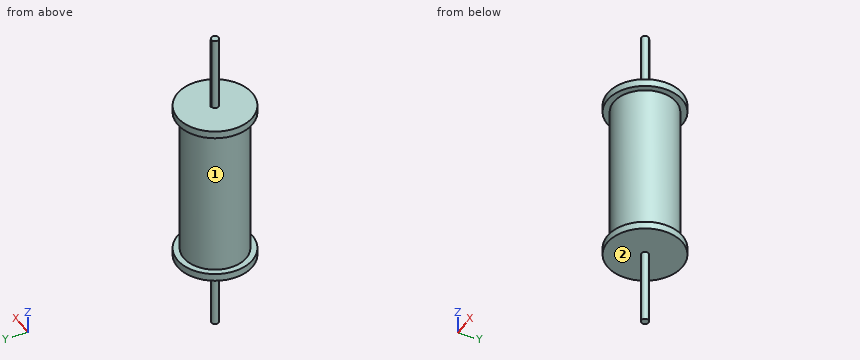
```python
from build123d import *

# Parameters (mm, degrees)
CROQUIS1_R              = 15
SALIENTE_EXTRUIR1_DEPTH = 3
SALIENTE_EXTRUIR2_DEPTH = 30
CROQUIS3_R              = 12.5
SALIENTE_EXTRUIR3_DEPTH = 61
SALIENTE_EXTRUIR4_START = 3
CROQUIS4_R              = 15
SALIENTE_EXTRUIR4_DEPTH = 3
SALIENTE_EXTRUIR5_START = 30
CROQUIS5_R              = 1.5
SALIENTE_EXTRUIR5_DEPTH = 30


with BuildPart() as part:
    # Croquis1 → Saliente-Extruir1 (new body)
    with BuildSketch(Plane.XY):
        Circle(CROQUIS1_R)
    extrude(amount=SALIENTE_EXTRUIR1_DEPTH)

    # Croquis2 → Saliente-Extruir2 (add)
    with BuildSketch(Plane.XY.offset(3)):
        with BuildLine():
            Line((-0.175, 1.489756692), (-0.175, 1.697953704))
            Line((-0.175, 1.697953704), (0.175, 1.697953704))
            Line((0.175, 1.697953704), (0.175, 1.489756692))
            ThreePointArc((0.175, 1.489756692), (0, -1.5), (-0.175, 1.489756692))
        make_face()
    extrude(amount=SALIENTE_EXTRUIR2_DEPTH)

    # Croquis3 → Saliente-Extruir3 (add)
    with BuildSketch(Plane(origin=(0, 0, 0), x_dir=(-1, 0, 0), z_dir=(0, 0, -1))):
        with Locations(Location((0, 0, 0), (0, 0, 180))):
            Circle(CROQUIS3_R)
    extrude(amount=SALIENTE_EXTRUIR3_DEPTH)

    # Croquis4 → Saliente-Extruir4 (add)
    with BuildSketch(Plane(origin=(0, 0, -61), x_dir=(-1, 0, 0), z_dir=(0, 0, -1)).offset(SALIENTE_EXTRUIR4_START)):
        with Locations(Location((0, 0, 0), (0, 0, 180))):
            Circle(CROQUIS4_R)
    extrude(amount=-SALIENTE_EXTRUIR4_DEPTH)

    # Croquis5 → Saliente-Extruir5 (add)
    with BuildSketch(Plane(origin=(0, 0, -64), x_dir=(-1, 0, 0), z_dir=(0, 0, -1)).offset(SALIENTE_EXTRUIR5_START)):
        Circle(CROQUIS5_R)
    extrude(amount=-SALIENTE_EXTRUIR5_DEPTH)


solid = part.part
```
Read the model definition and answer for the solid it produces. Units are mm, in the model's axes. Face numbers are marked on the shaded views. Coordinates: 2 decimals unless noted, no trailing zeros. Write each loop counter-clockwise with the first axis right and the second up, starting at its lowest first coordinate (ties: lowest second). Pieces come first, ordered by that corner, then holes. Notation, with made-up numbers: (75.25, 70.25) -> (103.25, 70.25) arc R5 ccw to (103.25, 76.25) -> close; hole circle Ø4 at (41.25, 72.25). An arc over 180 degrees is marked (long way). Answer as a JSON object with one key per item and string values.
Q1. The part is cut by section C-C on z = -5. Give the vertices of the cut face in (x, y).
The answers:
{"outline": "circle Ø25 at (0, 0)"}
Q2. The part is cut by section B-B on x = -9. Give the vertices of the cut face in (y, z).
The answers:
{"outline": "(-12, -64) -> (12, -64) -> (12, -61) -> (8.67, -61) -> (8.67, 0) -> (12, 0) -> (12, 3) -> (-12, 3) -> (-12, 0) -> (-8.67, 0) -> (-8.67, -61) -> (-12, -61) -> close"}
Q3. Flat-ended cylindrical pins translate along their axes: pin 1 Ø8 at (y, z) = (2, -12.5) entering from +X; pin 2 Ø5 at (x, y) = (-5, -2.5) entering from -Z; pin 3 Ø1.5 at (x, z) = (-5, -4.5) entering from -Y. Find the tip coordinate at first contact, or state that the pin passes through.
The answers:
{"pin 1": "stops at x = 12.5", "pin 2": "stops at z = -64", "pin 3": "stops at y = -11.76"}
Q4. Determine the mould class of the marked faces 1 and 2 for opening direction Z: pulls with the +Z half, pulls with the -Z half, needs draft (parallel to the pull), parting line crosses it, or undercut.
The answers:
{"face 1": "undercut", "face 2": "pulls with the -Z half"}
Q5. Consider line 1 (Z direction, x = -13.25, y = -3.5); line 2 (Z direction, x = -8.5, y = -2); line 3 (Y direction, x = -7.25, z = -49). Determine where each line is inside the solid, lowest interval first. Write a range as [from, to].
The answers:
{"line 1": "z = [-64, -61], [0, 3]", "line 2": "z = [-64, 3]", "line 3": "y = [-10.18, 10.18]"}
Q6. The part is cut by section A-A on y = 0. Give the vertices of the cut face in (x, z), then the cut area to 4 significant figures.
The answers:
{"outline": "(-15, -64) -> (-1.5, -64) -> (-1.5, -94) -> (1.5, -94) -> (1.5, -64) -> (15, -64) -> (15, -61) -> (12.5, -61) -> (12.5, 0) -> (15, 0) -> (15, 3) -> (1.5, 3) -> (1.5, 33) -> (-1.5, 33) -> (-1.5, 3) -> (-15, 3) -> (-15, 0) -> (-12.5, 0) -> (-12.5, -61) -> (-15, -61) -> close", "area": "1,885 mm2"}
